Part model, mm, in its own coordinate system. A direction names the side the tool comes from. Round coordinates to 2 decimals unless told otherwise and drop trailing zeros. Order: outer loops, then holes, each group sorted by start corner. A loop starts at its lowest first (then second) coordinate and runs counter-clockwise, first axis right, second up. Notation, with made-up numbers: M 76.25,-11 L 101.25,-11 A22 cw 101.25,27 Z; hole C 40,-31.75 d11. An arc over 180 degrees is marked long. Write each question's results on one line, items separated by ' | '. Start each with the question number.
1. Band-saw the part on A-A, the plane x = -22.5. List the corners of the cut face in (y, z), then the cut area to 3 significant figures.
2. Two-plate mould, pull along Y, no slides. Class faces 4 (the face through (-3.485, 17.394, -1.481)), 5 (the face through (-25.4, 1, -1)), 6 (the face through (-37, 11.112, -1)), 7 (the face through (-37, 23.812, -1)): +Y half, -Y half, draft (parallel to the pull), parting line (faces both ways), or undercut.
3. Band-saw the part on B-B, the plane z = -1.5. List the corners of the cut face in (x, y).
4. Drop flat-ended pins along their axis: pin 1 Ø1.5 at (y, z) = (1, -1.5) entering from +X; pin 2 Ø0.9 at (x, z) = (-1.5, -2) entering from -Y; pin 3 Ø5 at (x, y) = (-10, 31) entering from +Z; pin 4 Ø0.9 at (y, z) = (28.5, -2) entering from -X. Give the stop position or say it passes through.
5. Which spindle directions (+Z, -Z, +X, -X, +Y, -Y) get a long thin tool onto all of the face, cutting with end or side? Do faces 1 (the face through (-12.7, 1, -1)), 2 (the face through (-35.179, 5, -1)), 3 (the face through (-2.921, 5, -1)). Say none if no direction does.
6. Probe L1, parallel to Y at x = -24.5, z = -2.7; L2, parallel to X at y = 25, z = -0.85; L3, parallel to Y at x = -2, z = -1.5. List the from-to ranges inside material, lowest first. Write a range as [from, to].
7. Band-saw the part on C-C, the plane y = 5.5. List the corners of the cut face in (x, z).
```python
from build123d import *

# Parameters (mm, degrees)
SKETCH1_W             = 38.1
SKETCH1_H             = 38.1
BOSS_EXTRUDE1_DEPTH   = 2.921
SKETCH2_W             = 12.7
SKETCH2_H             = 2.921
CUT_EXTRUDE1_DEPTH    = 53.851725584
SKETCH3_W             = 2.921
SKETCH3_H             = 12.7
CUT_EXTRUDE2_DEPTH    = 53.851725584
F_6_CLEARANCE_HOLE2_D = 3.7973


with BuildPart() as part:
    # Sketch1 → Boss-Extrude1 (new body)
    with BuildSketch(Plane.XY):
        with Locations((-19.05, 17.4625)):
            Rectangle(SKETCH1_W, SKETCH1_H)
    extrude(amount=-BOSS_EXTRUDE1_DEPTH)

    # Sketch2 → Cut-Extrude1 (cut, through all)
    with BuildSketch(Plane.XY):
        with Locations((-19.05, 1.4605)):
            Rectangle(SKETCH2_W, SKETCH2_H)
    extrude(amount=-CUT_EXTRUDE1_DEPTH, mode=Mode.SUBTRACT)

    # Sketch3 → Cut-Extrude2 (cut, through all)
    with BuildSketch(Plane.XY):
        with Locations((-1.4605, 4.7625)):
            Rectangle(SKETCH3_W, SKETCH3_H)
        with Locations((-1.4605, 30.1625)):
            Rectangle(SKETCH3_W, SKETCH3_H)
        with Locations((-36.6395, 30.1625)):
            Rectangle(SKETCH3_W, SKETCH3_H)
        with Locations((-36.6395, 4.7625)):
            Rectangle(SKETCH3_W, SKETCH3_H)
    extrude(amount=-CUT_EXTRUDE2_DEPTH, mode=Mode.SUBTRACT)

    # #6 Clearance Hole2 (through all)
    with Locations(Plane.XY):
        with Locations((-1.5875, 17.4625), (-36.5125, 17.4625)):
            Hole(F_6_CLEARANCE_HOLE2_D / 2)


solid = part.part
```
Solution:
1) outline: M -1.59,-2.92 L 0,-2.92 L 0,0 L -1.59,0 Z; M 2.92,-2.92 L 36.51,-2.92 L 36.51,0 L 2.92,0 Z | area: 103 mm^2
2) face 4: undercut | face 5: undercut | face 6: -Y half | face 7: +Y half
3) outline: M -38.1,11.11 L -35.18,11.11 L -35.18,-1.59 L -2.92,-1.59 L -2.92,11.11 L 0,11.11 L 0,16.42 A1.9 cw long 0,18.5 L 0,23.81 L -2.92,23.81 L -2.92,36.51 L -35.18,36.51 L -35.18,23.81 L -38.1,23.81 L -38.1,18.5 A1.9 cw long -38.1,16.42 Z; hole M -25.4,0 L -12.7,0 L -12.7,2.92 L -25.4,2.92 Z
4) pin 1: x = -2.92 | pin 2: y = 11.11 | pin 3: z = 0 | pin 4: x = -35.18
5) face 1: +Z, -Z | face 2: +Z, -Z, -X, -Y | face 3: +Z, -Z, +X, -Y
6) L1: [-1.59, 0], [2.92, 36.51] | L2: [-35.18, -2.92] | L3: [11.11, 15.61], [19.32, 23.81]
7) outline: M -35.18,-2.92 L -2.92,-2.92 L -2.92,0 L -35.18,0 Z
